```python
from build123d import *

# Parameters (mm, degrees)
SKETCH1_R           = 76.5
SKETCH1_R_2         = 69.5
BOSS_EXTRUDE1_DEPTH = 7
SKETCH2_W           = 10.998336412
SKETCH2_H           = 3.996279506
BOSS_EXTRUDE2_DEPTH = 101
BOSS_EXTRUDE3_DEPTH = 7


with BuildPart() as part:
    # Sketch1 → Boss-Extrude1 (new body)
    with BuildSketch(Plane.XY):
        Circle(SKETCH1_R)
        Circle(SKETCH1_R_2, mode=Mode.SUBTRACT)
    extrude(amount=BOSS_EXTRUDE1_DEPTH)

    # Sketch2 → Boss-Extrude2 (add)
    with BuildSketch(Plane.XY.offset(7)):
        with Locations((0, 73.186602974)):
            Rectangle(SKETCH2_W, SKETCH2_H)
    extrude(amount=BOSS_EXTRUDE2_DEPTH)

    # Sketch3 → Boss-Extrude3 (add)
    with BuildSketch(Plane.XY.offset(108)):
        with BuildLine():
            Line((-18.119939766, 67.096332112), (-19.801444594, 73.89284669))
            ThreePointArc((-19.801444594, 73.89284669), (-0.302678458, 76.499401212), (19.216103117, 74.047223993))
            Line((19.216103117, 74.047223993), (17.850832513, 67.168428436))
            ThreePointArc((17.850832513, 67.168428436), (-0.139298774, 69.499860402), (-18.119939766, 67.096332112))
        make_face()
    extrude(amount=BOSS_EXTRUDE3_DEPTH)


solid = part.part
```
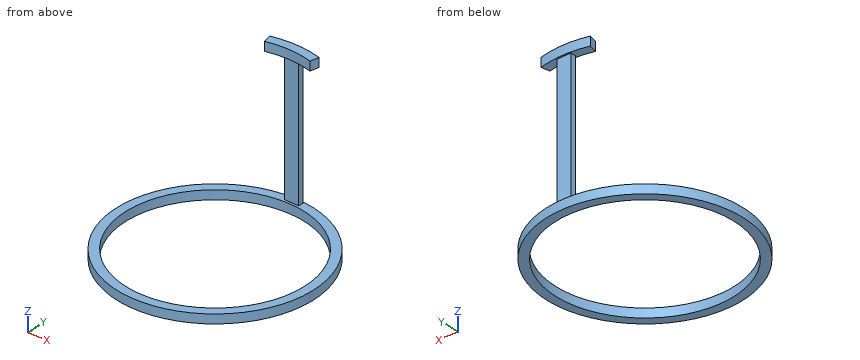
Build history of the part. All positions in model axes, mm. Coordinates: 2 decimals unless noted, no trailing zeros. Order: outer loops, then holes, each group sorted by start corner. A loop starts at its lowest first (then second) coordinate and runs counter-clockwise, first axis right, second up. Notation, with made-up numbers: M -35,19.5 L 13,19.5 A31 ccw 13,47.5 Z; hole C 61.5,-21.5 d7. An arc over 180 degrees is marked long. One line per question, with ' | ' between items. Start each with the question number.
1. Flat gauge pins, fed straight in: P1, Ø12, axis at x = 0.5, z = 45, coming from the +Y side; P2, Ø12, axis at x = -41.5, z = 12.5, coming from the +Y side; P3, Ø9, axis at x = -0.5, z = 58.5, coming from the -Y side. Where does each tip first touch, or does it go through?
2. Cut at B-B (x = 0). Write the cut outline in (y, z), plus the area to 3 significant figures.
3. Cut at C-C (y = 18). Write the cut outline in (x, z).
4. Cut at D-D (z = 41.5). Write the cut outline in (x, y), plus the area to 3 significant figures.
5. Wall check: line 1 along Y through (x, z) = (0, 2); line 2 along Z through (x, y) = (-66.5, -25); line 3 along Y through (x, z) = (3, 99). Give the ranges that are in metal, low to high. Write a range as [from, to].
6. Cut at A-A (y = 0). Write the cut outline in (x, z), plus the area to 3 significant figures.
The answers:
1) P1: stops at y = 75.18 | P2: stops at y = 65.75 | P3: stops at y = 71.19
2) outline: M -76.5,0 L -69.5,0 L -69.5,7 L -76.5,7 Z; M 69.5,0 L 76.5,0 L 76.5,7 L 75.18,7 L 75.18,108 L 76.5,108 L 76.5,115 L 69.5,115 L 69.5,108 L 71.19,108 L 71.19,7 L 69.5,7 Z | area: 551 mm2
3) outline: M -74.35,0 L -67.13,0 L -67.13,7 L -74.35,7 Z; M 67.13,0 L 74.35,0 L 74.35,7 L 67.13,7 Z
4) outline: M -5.5,71.19 L 5.5,71.19 L 5.5,75.18 L -5.5,75.18 Z | area: 44.0 mm2
5) line 1: y = [-76.5, -69.5], [69.5, 76.5] | line 2: z = [0, 7] | line 3: y = [71.19, 75.18]
6) outline: M -76.5,0 L -69.5,0 L -69.5,7 L -76.5,7 Z; M 69.5,0 L 76.5,0 L 76.5,7 L 69.5,7 Z | area: 98.0 mm2
